from build123d import *

# Parameters (mm, degrees)
F0_R     = 27.5
F1_DEPTH = 2
F2_R     = 6.5
F2_R_2   = 1.5
F3_DEPTH = 2
F4_R     = 1.5
F5_DEPTH = 2
F7_DEPTH = 175


with BuildPart() as f1:
    # F0 (on Front) → F1 (new body)
    with BuildSketch(Plane.XZ):
        Polygon((44, 44), (-44, 44), (-66, 34), (-87.5, 2), (-87.5, -55), (87.5, -55), (87.5, 2), (66, 34), align=None)
        Circle(F0_R, mode=Mode.SUBTRACT)
    extrude(amount=F1_DEPTH)

    # F2 (on face) → F3 (cut, through all)
    with BuildSketch(Plane.XZ.offset(2)):
        with Locations((50, 16)):
            Circle(F2_R)
        with Locations((61.746158, 20.275252)):
            Circle(F2_R_2)
        with Locations((38.253842, 11.724748)):
            Circle(F2_R_2)
        with Locations((-38.253842, 11.724748)):
            Circle(F2_R_2)
        with Locations((-61.746158, 20.275252)):
            Circle(F2_R_2)
        with Locations((-50, 16)):
            Circle(F2_R)
    extrude(amount=-F3_DEPTH, mode=Mode.SUBTRACT)

    # F4 (on face) → F5 (cut, through all)
    with BuildSketch(Plane.XZ.offset(2)):
        with Locations((-31.5, -45)):
            Circle(F4_R)
        with Locations((31.5, -45)):
            Circle(F4_R)
        with Locations((76, -30)):
            Circle(F4_R)
        with Locations((72.5, 8)):
            Circle(F4_R)
        with Locations((40.5, 37)):
            Circle(F4_R)
        with Locations((-40.5, 37)):
            Circle(F4_R)
        with Locations((-76, -30)):
            Circle(F4_R)
        with Locations((-72.5, 8)):
            Circle(F4_R)
    extrude(amount=-F5_DEPTH, mode=Mode.SUBTRACT)

    # F6 (on face) → F7 (join, through all)
    with BuildSketch(Plane.YZ.offset(87.5)):
        Polygon((0, -52.690599), (0, -55), (18.186533, -44.5), (17.186533, -42.767949), align=None)
    extrude(amount=-F7_DEPTH)


solid = f1.part
The listing builds one solid part. Answer for the finished solid, in the listing's coordinates (mm). A direction names the side the tool comes from. Coordinates: 2 decimals unless noted, no trailing zeros. Write each loop counter-clockwise with the first axis right and the second up, starting at its lowest first coordinate (ties: lowest second). Pieces come first, ordered by that corner, then holes. Notation, with made-up numbers: M -36,-12 L -15,-12 A21 ccw -15,10 Z; hole C -24,6 d1. An arc over 180 degrees is marked long. Put each result on its own line as item: value. Start each with the question number.
1. A cutting plane is placed at B-B on x = -14. Write down the section's boundary in (y, z).
2. Which of the six approach directions +Z, -Z, +X, -X, +Y, -Y give full straight-line access (tool end or side, diameter ignored) to faces 4 (the flat face through (1.22, 8.71, -47.66)), 5 (the flat face through (-55, -1, 39))?
3. For a pull along X with two mould halves and no side action, classify faces 1 (the cylindrical face through (43.506, -1.014, 16.286)), 2 (the flat face through (18, -2, -27)), 3 (the flat face through (55, -1, 39)) as pulls with the +X half, pulls with the -X half, needs draft (parallel to the pull), parting line crosses it, or undercut.
4. A cutting plane is placed at D-D on x = 50. Write down the section's boundary in (y, z), then the cut area to 3 significant figures.
5. A cutting plane is placed at C-C on z = 16. Write down the section's boundary in (x, y), then the cut area to 3 significant figures.
6. Flat-ended cylindrical pins translate along their axes: P1, Ø1.8, axis at x = -40.5, z = 37, coming from the -Y side; P2, Ø3.5, axis at x = 72.5, z = 8, coming from the +Y side; P3, Ø10, axis at x = 10.5, y = 8, coming from the -Z side; P4, Ø12, axis at x = -59, y = 8.5, coming from the +Z side. Find the tip coordinate at first contact, or state that the pin passes through.
7. Consider line 1 (Y direction, x = -55.5, z = -33); line 2 (Z direction, x = -76, y = -1.45); line 3 (Z direction, x = 72.5, y = -0.95). Determine where each line is inside the solid, lowest interval first. Write a range as from..to.
8. A cutting plane is placed at A-A on z = 0. Write down the section's boundary in (x, y), then the cut area to 3 significant figures.
Resolved:
1. outline: M -2,-55 L 0,-55 L 18.19,-44.5 L 17.19,-42.77 L 0,-52.69 L 0,-23.67 L -2,-23.67 Z; M -2,23.67 L 0,23.67 L 0,44 L -2,44 Z
2. face 4: +Z, +X, -X
2. face 5: +Z, -X, +Y, -Y
3. face 1: undercut
3. face 2: needs draft
3. face 3: pulls with the +X half
4. outline: M -2,-55 L 0,-55 L 18.19,-44.5 L 17.19,-42.77 L 0,-52.69 L 0,9.5 L -2,9.5 Z; M -2,22.5 L 0,22.5 L 0,41.27 L -2,41.27 Z
4. area: 207 mm2
5. outline: M -78.09,-2 L -56.5,-2 L -56.5,0 L -78.09,0 Z; M -43.5,-2 L -22.37,-2 L -22.37,0 L -43.5,0 Z; M 22.37,-2 L 43.5,-2 L 43.5,0 L 22.37,0 Z; M 56.5,-2 L 78.09,-2 L 78.09,0 L 56.5,0 Z
5. area: 171 mm2
6. P1: passes through
6. P2: stops at y = 0
6. P3: stops at z = -53.27
6. P4: stops at z = -44.32
7. line 1: y = -2..0
7. line 2: z = -55..-31.5, -28.5..19.12
7. line 3: z = -55..6.5, 9.5..24.33
8. outline: M -87.5,-2 L -27.5,-2 L -27.5,0 L -87.5,0 Z; M 27.5,-2 L 87.5,-2 L 87.5,0 L 27.5,0 Z
8. area: 240 mm2
